Study the drawing (mm; zero at the part's minimum x, y, z) and answer. A direction names the side the tool comes from. Give positions to 0.01 mm unless a question says otherwise; leave off trailing zeros. Loops run counter-clockwise (first coordinate to the right, second up) from the corner with the lowest first, then second, coordinate; pieces in that order, holes last. Notation, with made-up numbers: (14.25, -1.5) - (53.25, -1.5) arc R22 cw to (53.25, 27.5) - close; hole circle Ø11 at (-31.75, -34.5). An arc over 180 degrees is marked (long way). Write item = value, one per line. Start each with the question number.
1) The part is cut by section B-B on x = 23.8. Write down the section's boundary in (y, z).
2) The part is cut by section D-D on x = 13.8. Write down the section's boundary in (y, z), plus the area to 3 significant figures.
3) Flat-ended cylindrical pins translate along their axes: P1, Ø3, axis at y = 9.5, z = 1.5, coming from the -X side; P2, Ø3.5, axis at x = 17.5, y = 2, coming from the +Z side. Find the tip coordinate at first contact, or state that the pin passes through.
4) The part is cut by section A-A on z = 6.6. Write down the section's boundary in (x, y).
5) Consider probe 1 along Z at (x, y) = (23.8, 8); probe 2 along X at (y, z) = (10, 5.5); probe 3 along X at (y, z) = (1.5, 8.5). Determine where each line is inside the solid, lowest interval first.
6) The part is cut by section C-C on y = 2.5. Write down the section's boundary in (x, z).
7) The mould has two halves that part along Z. Classify the marked faces 3, 4 and 5: +Z half, -Z half, draft (parallel to the pull), parting line (faces both ways), or undercut.
8) Which of the six approach directions +Z, -Z, +X, -X, +Y, -Y give full straight-line access (tool end or side, diameter ignored) to the marked faces 1 and 2?
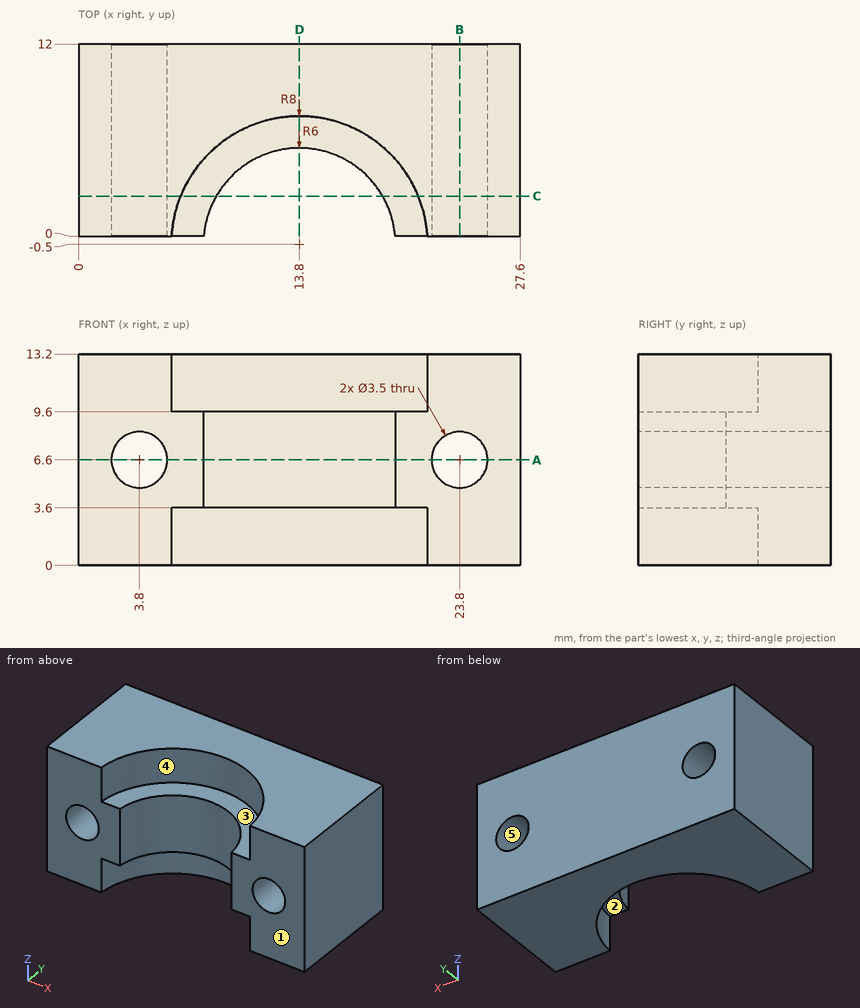
Answer below:
q1.outline = (0, 0) - (12, 0) - (12, 4.85) - (0, 4.85) - close; (0, 8.35) - (12, 8.35) - (12, 13.2) - (0, 13.2) - close
q2.outline = (5.5, 3.6) - (7.5, 3.6) - (7.5, 0) - (12, 0) - (12, 13.2) - (7.5, 13.2) - (7.5, 9.6) - (5.5, 9.6) - close
q2.area = 71.4 mm2
q3.P1 = 0
q3.P2 = 9.6
q4.outline = (0, 0) - (2.05, 0) - (2.05, 12) - (0, 12) - close; (5.55, 0) - (7.82, 0) arc R6 cw to (19.78, 0) - (22.05, 0) - (22.05, 12) - (5.55, 12) - close; (25.55, 0) - (27.6, 0) - (27.6, 12) - (25.55, 12) - close
q5.probe_1 = 0 to 4.85, 8.35 to 13.2
q5.probe_2 = 0 to 2.44, 5.16 to 22.44, 25.16 to 27.6
q5.probe_3 = 0 to 8.14, 19.46 to 27.6
q6.outline = (0, 0) - (6.38, 0) - (6.38, 3.6) - (8.6, 3.6) - (8.6, 9.6) - (6.38, 9.6) - (6.38, 13.2) - (0, 13.2) - close; (19, 3.6) - (21.22, 3.6) - (21.22, 0) - (27.6, 0) - (27.6, 13.2) - (21.22, 13.2) - (21.22, 9.6) - (19, 9.6) - close; hole circle Ø3.5 at (3.8, 6.6); hole circle Ø3.5 at (23.8, 6.6)
q7.face_3 = +Z half
q7.face_4 = draft
q7.face_5 = undercut
q8.face_1 = +Z, -Z, +X, -X, -Y
q8.face_2 = -Z, -Y
